from build123d import *

# Parameters (mm, degrees)
SKETCH1_W           = 64
SKETCH1_H           = 42
BOSS_EXTRUDE1_DEPTH = 2
FILLET1_R           = 8
BOSS_EXTRUDE2_DEPTH = 1.2
SKETCH3_W           = 6
SKETCH3_H           = 25.2
CUT_EXTRUDE1_DEPTH  = 1.2
SKETCH4_R           = 2
BOSS_EXTRUDE3_DEPTH = 7.5
SKETCH5_R           = 0.8
CUT_EXTRUDE2_DEPTH  = 5
SKETCH6_R           = 5.1
SKETCH6_R_2         = 1.25
SKETCH6_W           = 6
SKETCH6_H           = 4
CUT_EXTRUDE3_DEPTH  = 40.003204997


with BuildPart() as part:
    # Sketch1 → Boss-Extrude1 (new body)
    with BuildSketch(Plane.XY):
        Rectangle(SKETCH1_W, SKETCH1_H)
    extrude(amount=BOSS_EXTRUDE1_DEPTH)

    # Fillet1
    fillet1_edges = [part.edges().sort_by_distance(p)[0] for p in [
        (-32, 21, 1),
        (32, 21, 1),
        (32, -21, 1),
        (-32, -21, 1),
    ]]
    fillet(fillet1_edges, radius=FILLET1_R)

    # Sketch2 → Boss-Extrude2 (add)
    with BuildSketch(Plane.XY.offset(2)):
        with BuildLine():
            Line((-24, 19.2), (24, 19.2))
            ThreePointArc((24, 19.2), (28.384062043, 17.384062043), (30.2, 13))
            Line((30.2, 13), (30.2, -13))
            ThreePointArc((30.2, -13), (28.384062043, -17.384062043), (24, -19.2))
            Line((24, -19.2), (-24, -19.2))
            ThreePointArc((-24, -19.2), (-28.384062043, -17.384062043), (-30.2, -13))
            Line((-30.2, -13), (-30.2, 13))
            ThreePointArc((-30.2, 13), (-28.384062043, 17.384062043), (-24, 19.2))
        make_face()
        with BuildLine():
            Line((-24, 17.7), (24, 17.7))
            ThreePointArc((24, 17.7), (27.323401872, 16.323401872), (28.7, 13))
            Line((28.7, 13), (28.7, -13))
            ThreePointArc((28.7, -13), (27.323401872, -16.323401872), (24, -17.7))
            Line((24, -17.7), (-24, -17.7))
            ThreePointArc((-24, -17.7), (-27.323401872, -16.323401872), (-28.7, -13))
            Line((-28.7, -13), (-28.7, 13))
            ThreePointArc((-28.7, 13), (-27.323401872, 16.323401872), (-24, 17.7))
        make_face(mode=Mode.SUBTRACT)
    extrude(amount=BOSS_EXTRUDE2_DEPTH)

    # Sketch3 → Cut-Extrude1 (cut)
    with BuildSketch(Plane(origin=(0, 0, 2), x_dir=(-1, 0, 0), z_dir=(0, 0, -1))):
        with Locations((-30, 0)):
            Rectangle(SKETCH3_W, SKETCH3_H)
    extrude(amount=-CUT_EXTRUDE1_DEPTH, mode=Mode.SUBTRACT)

    # Sketch4 → Boss-Extrude3 (add)
    with BuildSketch(Plane.XY.offset(2)):
        with Locations((-6, 15)):
            Circle(SKETCH4_R)
        with Locations((24, 15)):
            Circle(SKETCH4_R)
        with Locations(Location((24, -15, 0), (0, 0, 180))):
            Circle(SKETCH4_R)
        with Locations(Location((-6, -15, 0), (0, 0, 180))):
            Circle(SKETCH4_R)
    extrude(amount=BOSS_EXTRUDE3_DEPTH)

    # Sketch5 → Cut-Extrude2 (cut)
    with BuildSketch(Plane.XY.offset(9.5)):
        with Locations((24, 15)):
            Circle(SKETCH5_R)
    cut_extrude2 = extrude(amount=-CUT_EXTRUDE2_DEPTH, mode=Mode.SUBTRACT)

    # Sketch-Pattern1: Cut-Extrude2 at 3 more places
    with Locations((-30, 0, 0), (-30, -30, 0), (0, -30, 0)):
        add(cut_extrude2, mode=Mode.SUBTRACT)

    # Sketch6 → Cut-Extrude3 (cut, through all)
    with BuildSketch(Plane.XY.offset(2)):
        with Locations((-19, 0)):
            Circle(SKETCH6_R)
        with Locations((8, -15)):
            Circle(SKETCH6_R_2)
        with Locations((2, -15)):
            Rectangle(SKETCH6_W, SKETCH6_H)
    extrude(amount=-CUT_EXTRUDE3_DEPTH, mode=Mode.SUBTRACT)


solid = part.part
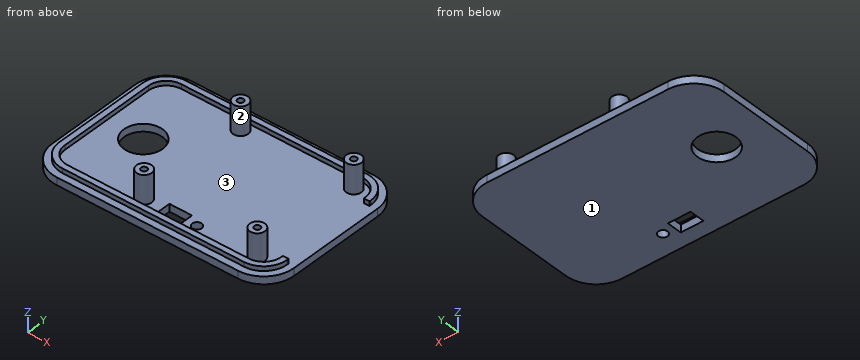
Check sheet for the modelled part. Datum: model origin and axes. Units: mm. Face numbers are marked on the shaded views. Round coordinates to 2 decimals unless told otherwise and drop trailing zeros. Order: outer loops, then holes, each group sorted by start corner. A loop starts at its lowest first (then second) coordinate and runs counter-clockwise, first axis right, second up.
Q1. Cross-section at D-D, the plane z = 1. Enter the section's corners in (x, y).
Filled sheet:
outline: (-32, -13) arc R8 ccw to (-24, -21) - (24, -21) arc R8 ccw to (32, -13) - (32, 13) arc R8 ccw to (24, 21) - (-24, 21) arc R8 ccw to (-32, 13) - close; hole circle Ø10.2 at (-19, 0); hole (-1, -17) - (5, -17) - (5, -13) - (-1, -13) - close; hole circle Ø2.5 at (8, -15)
Q2. Cross-section at A-A, the plane z = 6. Enter the section's corners in (x, y).
Filled sheet:
outline: circle Ø4 at (-6, -15); circle Ø4 at (-6, 15); circle Ø4 at (24, -15); circle Ø4 at (24, 15); hole circle Ø1.6 at (-6, -15); hole circle Ø1.6 at (-6, 15); hole circle Ø1.6 at (24, -15); hole circle Ø1.6 at (24, 15)
Q3. Draft check along Y on the marked faces 1, 2 and 3. Enter one of: pulls with the +Y half, pulls with the -Y half, needs draft (parallel to the pull), parting line crosses it, or undercut.
Filled sheet:
face 1: needs draft
face 2: undercut
face 3: undercut
Q4. Depth check by flat-ended pin: P1, Ø1, axis at y = -15.5, z = 1, coming from the +X side; P2, Ø2, axis at x = 1.5, y = 11.5, coming from the -Z side; P3, Ø0.8, axis at x = -6, y = -15, coming from the +Z side; P4, Ø1.3, axis at x = 29.5, z = 2.5, coming from the +Y side. Enter the tip coordinate at first touch or a pass-through.
Filled sheet:
P1: stops at x = 31.75
P2: stops at z = 0
P3: stops at z = 4.5
P4: stops at y = 19.18
Q5. Scan lines: L1, parallel to Y at x = -6, z = 8.15; L2, parallel to Y at x = 8, z = 1.65; L3, parallel to Y at x = 20.5, z = 2.75. Record each from-to range of solid material in increasing order.
Filled sheet:
L1: y = -17 to -15.8, -14.2 to -13, 13 to 14.2, 15.8 to 17
L2: y = -21 to -16.25, -13.75 to 21
L3: y = -19.2 to -17.7, 17.7 to 19.2
Q6. Cross-section at C-C, the plane y = 0. Enter the section's corners in (x, z), plus the area to 3 significant figures.
Filled sheet:
outline: (-32, 0) - (-24.1, 0) - (-24.1, 2) - (-28.7, 2) - (-28.7, 3.2) - (-30.2, 3.2) - (-30.2, 2) - (-32, 2) - close; (-13.9, 0) - (32, 0) - (32, 2) - (-13.9, 2) - close
area: 109 mm2
Q7. Cross-section at B-B, the plane x = 8. Enter the section's corners in (y, z), plus the area to 3 significant figures.
Filled sheet:
outline: (-21, 0) - (-16.25, 0) - (-16.25, 2) - (-17.7, 2) - (-17.7, 3.2) - (-19.2, 3.2) - (-19.2, 2) - (-21, 2) - close; (-13.75, 0) - (21, 0) - (21, 2) - (19.2, 2) - (19.2, 3.2) - (17.7, 3.2) - (17.7, 2) - (-13.75, 2) - close
area: 82.6 mm2
